```python
from build123d import *

# Parameters (mm, degrees)
F0_W      = 55
F0_H      = 40
F1_DEPTH  = 2
F3_R      = 5.08
F4_R      = 5.08
F5_R      = 5.08
F6_R      = 5.08
F8_R      = 1.5
F9_DEPTH  = 25.4
F10_W     = 10
F10_H     = 4
F11_DEPTH = 25.4


with BuildPart() as f1:
    # F0 (on Top) → F1 (new body)
    with BuildSketch(Plane.XY):
        with Locations((27.5, 20)):
            Rectangle(F0_W, F0_H)
    extrude(amount=F1_DEPTH)

    # F3
    f3_edges = [f1.edges().sort_by_distance(p)[0] for p in [
        (55, 0, 1),
    ]]
    fillet(f3_edges, radius=F3_R)

    # F4
    f4_edges = [f1.edges().sort_by_distance(p)[0] for p in [
        (55, 40, 1),
    ]]
    fillet(f4_edges, radius=F4_R)

    # F5
    f5_edges = [f1.edges().sort_by_distance(p)[0] for p in [
        (0, 40, 1),
    ]]
    fillet(f5_edges, radius=F5_R)

    # F6
    f6_edges = [f1.edges().sort_by_distance(p)[0] for p in [
        (0, 0, 1),
    ]]
    fillet(f6_edges, radius=F6_R)

    # F8 (on offset) → F9 (cut)
    with BuildSketch(Plane.XY.offset(2)):
        with Locations((50, 5)):
            Circle(F8_R)
        with Locations((47.1494022449, 8.3385913854)):
            Circle(F8_R)
        with Locations((47.1494022449, 31.6614086146)):
            Circle(F8_R)
        with Locations((50, 35)):
            Circle(F8_R)
        with Locations((7.8505977551, 31.6614086146)):
            Circle(F8_R)
        with Locations((5, 35)):
            Circle(F8_R)
        with Locations((7.8505977551, 8.3385913854)):
            Circle(F8_R)
        with Locations((5, 5)):
            Circle(F8_R)
    extrude(amount=-F9_DEPTH, mode=Mode.SUBTRACT)

    # F10 (on face) → F11 (cut)
    with BuildSketch(Plane.XY.offset(2)):
        with BuildLine():
            Line((20, 17.5), (20, 22.5))
            Line((20, 22.5), (20.8850657517, 22.5))
            add(Edge.make_bspline(
                [(20.8850657517, 22.5), (14.9931568267, 23.0368228686), (14.9931568267, 20)],
                knots=[4.5346839474, 4.5346839474, 4.5346839474, 6.2831853072, 6.2831853072, 6.2831853072], degree=2, weights=[1, 0.6415718139, 1]))
            add(Edge.make_bspline(
                [(14.9931568267, 20), (14.9931568267, 16.9631771314), (20.8850657517, 17.5)],
                knots=[0, 0, 0, 1.7485013598, 1.7485013598, 1.7485013598], degree=2, weights=[1, 0.6415718139, 1]))
            Line((20.8850657517, 17.5), (20, 17.5))
        make_face()
        with BuildLine():
            Line((20.8850657517, 22.5), (20, 22.5))
            Line((20, 22.5), (20, 17.5))
            Line((20, 17.5), (20.8850657517, 17.5))
            add(Edge.make_bspline(
                [(20.8850657517, 17.5), (25.0068431733, 17.8755428686), (25.0068431733, 20), (25.0068431733, 22.1244571314), (20.8850657517, 22.5)],
                knots=[1.7485013598, 1.7485013598, 1.7485013598, 3.1415926536, 3.1415926536, 4.5346839474, 4.5346839474, 4.5346839474], degree=2, weights=[1, 0.767062975, 1, 0.767062975, 1]))
        make_face()
        with BuildLine():
            Line((35, 22.5), (20.8850657517, 22.5))
            add(Edge.make_bspline(
                [(20.8850657517, 17.5), (25.0068431733, 17.8755428686), (25.0068431733, 20), (25.0068431733, 22.1244571314), (20.8850657517, 22.5)],
                knots=[1.7485013598, 1.7485013598, 1.7485013598, 3.1415926536, 3.1415926536, 4.5346839474, 4.5346839474, 4.5346839474], degree=2, weights=[1, 0.767062975, 1, 0.767062975, 1]))
            Line((20.8850657517, 17.5), (35, 17.5))
            Line((35, 17.5), (35, 22.5))
        make_face()
        with Locations((30, 25.5)):
            Rectangle(F10_W, F10_H)
        Polygon((25, 23.5), (25, 27.5), (20, 23.5), align=None)
        Polygon((20, 16.5094), (25, 12.5094), (25, 16.5094), align=None)
        with Locations((30, 14.5094)):
            Rectangle(F10_W, F10_H)
        with BuildLine():
            Line((43.6482731998, 25.5), (38, 27.5))
            ThreePointArc((38, 27.5), (36.4781820371, 25.5), (38, 23.5))
            Line((38, 23.5), (43.6482731998, 25.5))
        make_face()
        with BuildLine():
            ThreePointArc((38, 16.5094), (36.4781820371, 14.5094), (38, 12.5094))
            Line((38, 12.5094), (43.6482731998, 14.5094))
            Line((43.6482731998, 14.5094), (38, 16.5094))
        make_face()
    extrude(amount=-F11_DEPTH, mode=Mode.SUBTRACT)


solid = f1.part
```
For this review, take the finished solid that the model builds, in its own axes (mm). A direction names the side the tool comes from. Coordinates: 2 decimals unless noted, no trailing zeros. Write each loop counter-clockwise with the first axis right and the second up, starting at its lowest first coordinate (ties: lowest second). Pieces come first, ordered by that corner, then holes. Notation, with made-up numbers: (22.5, 52) -> (69.5, 52) arc R22 ccw to (69.5, 87) -> close; hole circle Ø4 at (-35, 48.25). An arc over 180 degrees is marked (long way). Put each result on its own line as item: value.
Q1. Take a section at A-A, the plane x = 32.5. State the section outline as (y, z) points.
From the geometry:
outline: (0, 0) -> (12.51, 0) -> (12.51, 2) -> (0, 2) -> close; (16.51, 0) -> (17.5, 0) -> (17.5, 2) -> (16.51, 2) -> close; (22.5, 0) -> (23.5, 0) -> (23.5, 2) -> (22.5, 2) -> close; (27.5, 0) -> (40, 0) -> (40, 2) -> (27.5, 2) -> close
Q2. Wall thickness on L1, parallel to Y at x = 5, z = 1.15; L2, parallel to X at y = 8, z = 1.45; L3, parallel to Y at x = 47, z = 1.9: over which ranges is each line inside the solid? List them lowest first.
From the geometry:
L1: y = 0 to 3.5, 6.5 to 33.5, 36.5 to 40
L2: x = 0 to 6.39, 9.31 to 45.69, 48.61 to 55
L3: y = 0 to 6.85, 9.83 to 30.17, 33.15 to 40
Q3. Take a section at B-B, the plane y = 13.5. State the section outline as (x, z) points, then the cut area to 3 significant figures.
From the geometry:
outline: (0, 0) -> (23.76, 0) -> (23.76, 2) -> (0, 2) -> close; (35, 0) -> (36.74, 0) -> (36.74, 2) -> (35, 2) -> close; (40.8, 0) -> (55, 0) -> (55, 2) -> (40.8, 2) -> close
area: 79.4 mm2
Q4. Tool access review of faces 4 (the flat face through (35, 25, 1)), 5 (the flat face through (21, 25, 0)): name each direction out of +Z, -Z, +X, -X, +Y, -Y from which nothing blocks a thin tool from reaching the whole face with its end or side.
From the geometry:
face 4: +Z, -Z
face 5: -Z, +X, -X, +Y, -Y
Q5. Take a section at C-C, the plane x = 7.5. State the section outline as (y, z) points, then the cut area to 3 significant figures.
From the geometry:
outline: (0, 0) -> (6.88, 0) -> (6.88, 2) -> (0, 2) -> close; (9.8, 0) -> (30.2, 0) -> (30.2, 2) -> (9.8, 2) -> close; (33.12, 0) -> (40, 0) -> (40, 2) -> (33.12, 2) -> close
area: 68.3 mm2
Q6. The part is to be moulded in two halves that separate along Y. For faces 1 (the cylindrical face through (1.449, 1.528, 1.014)), 2 (the flat face through (40.785, 24.486, 1.014)), 3 (the flat face through (27, 40, 1)), say which applies: +Y half, -Y half, draft (parallel to the pull), parting line (faces both ways), or undercut.
From the geometry:
face 1: -Y half
face 2: undercut
face 3: +Y half
Q7. Take a section at D-D, the plane z = 1.6. Count the separate pieces of the cut face and the enclosed holes in it, then the cut area to 3 significant figures.
From the geometry:
separate pieces: 1
enclosed holes: 13
area: 1,890 mm2
